```python
from build123d import *

# Parameters (mm, degrees)
CUT_EXTRUDE1_DEPTH      = 296.465734054
CUT_EXTRUDE1_DEPTH_BACK = 296.465734054
SKETCH2_R               = 6.1


with BuildPart() as part:
    # Sketch1 → Revolve1 (revolve)
    with BuildSketch(Plane.XY):
        Polygon((-21.25, -80), (-21.25, -67), (-17.5, -67), (-17.5, 67), (-21.25, 67), (-21.25, 80), (-42.5, 80), (-125, 80), (-125, 70), (-125, -70), (-180, -70), (-180, -80), (-42.5, -80), align=None)
    revolve(axis=Axis((0, 80, 0), (0, -1, 0)))

    # Sketch2 → Cut-Extrude1 (cut, two sides: drawn at the far end of the back side and taken through both)
    with BuildSketch(Plane(origin=(0, -70, 0), x_dir=(1, 0, 0), z_dir=(0, 1, 0)).offset(-CUT_EXTRUDE1_DEPTH_BACK)):
        with Locations(Location((0, 150, 0), (0, 0, 270))):
            Circle(SKETCH2_R)
        with Locations(Location((57.402514855, 138.581929877, 0), (0, 0, 270))):
            Circle(SKETCH2_R)
        with Locations(Location((106.066017178, 106.066017178, 0), (0, 0, 270))):
            Circle(SKETCH2_R)
        with Locations(Location((138.581929877, 57.402514855, 0), (0, 0, 270))):
            Circle(SKETCH2_R)
        with Locations(Location((150, 0, 0), (0, 0, 270))):
            Circle(SKETCH2_R)
        with Locations(Location((138.581929877, -57.402514855, 0), (0, 0, 270))):
            Circle(SKETCH2_R)
        with Locations(Location((106.066017178, -106.066017178, 0), (0, 0, 270))):
            Circle(SKETCH2_R)
        with Locations(Location((57.402514855, -138.581929877, 0), (0, 0, 270))):
            Circle(SKETCH2_R)
        with Locations(Location((0, -150, 0), (0, 0, 270))):
            Circle(SKETCH2_R)
        with Locations(Location((-57.402514855, -138.581929877, 0), (0, 0, 270))):
            Circle(SKETCH2_R)
        with Locations(Location((-106.066017178, -106.066017178, 0), (0, 0, 270))):
            Circle(SKETCH2_R)
        with Locations(Location((-138.581929877, -57.402514855, 0), (0, 0, 270))):
            Circle(SKETCH2_R)
        with Locations(Location((-150, 0, 0), (0, 0, 270))):
            Circle(SKETCH2_R)
        with Locations(Location((-138.581929877, 57.402514855, 0), (0, 0, 270))):
            Circle(SKETCH2_R)
        with Locations(Location((-106.066017178, 106.066017178, 0), (0, 0, 270))):
            Circle(SKETCH2_R)
        with Locations(Location((-57.402514855, 138.581929877, 0), (0, 0, 270))):
            Circle(SKETCH2_R)
    extrude(amount=CUT_EXTRUDE1_DEPTH + CUT_EXTRUDE1_DEPTH_BACK, mode=Mode.SUBTRACT)


solid = part.part
```
Read the model definition and answer for the solid it produces. Units are mm, in the model's axes. A direction names the side the tool comes from. Give positions to 0.01 mm unless a question says otherwise; leave off trailing zeros. Write each loop counter-clockwise with the first axis right and the second up, starting at its lowest first coordinate (ties: lowest second). Pieces come first, ordered by that corner, then holes. Notation, with made-up numbers: (75, 34) -> (114, 34) arc R25 ccw to (114, 52) -> close; hole circle Ø7 at (-25, 17). An arc over 180 degrees is marked (long way). Answer in a Markdown table with one row per item.
1) Determine the mould class of faces 4 (the cylindrical face through (16.863, 73.591, 12.93)), 5 (the cylindrical face through (144.045, -75.07, -1.322)), 6 (the flat face through (-2, 80, 26)), 7 (the cylindrical face through (-83.06, -75.07, 159.69)) for opening direction X: released by +X, released by -X, zero draft, split by the parting line, or undercut.
Results list:
| item | result |
|---|---|
| face 4 | undercut |
| face 5 | undercut |
| face 6 | zero draft |
| face 7 | split by the parting line |
2) Section A-A on z = 0 is taken. Give the vertices of the cut face in (x, y), plus the area to 3 significant figures.
Results list:
| item | result |
|---|---|
| outline | (-180, -80) -> (-156.1, -80) -> (-156.1, -70) -> (-180, -70) -> close; (-143.9, -80) -> (-21.25, -80) -> (-21.25, -67) -> (-17.5, -67) -> (-17.5, 67) -> (-21.25, 67) -> (-21.25, 80) -> (-125, 80) -> (-125, -70) -> (-143.9, -70) -> close; (17.5, -67) -> (21.25, -67) -> (21.25, -80) -> (143.9, -80) -> (143.9, -70) -> (125, -70) -> (125, 80) -> (21.25, 80) -> (21.25, 67) -> (17.5, 67) -> close; (156.1, -80) -> (180, -80) -> (180, -70) -> (156.1, -70) -> close |
| area | 35,100 mm^2 |
3) A tool of negligible diameter and unlimited length cuts with its end or side. For faces 1 (the flat face through (-3, -67, -17.4)), 2 (the flat face through (-123, -70, 37)), 3 (the cylindrical face through (0.268, -75.07, -156.094)), from which of +Z, -Z, +X, -X, +Y, -Y can it reach the whole face along a straight path? Write none if from no direction.
Results list:
| item | result |
|---|---|
| face 1 | -Y |
| face 2 | +Y |
| face 3 | +Y, -Y |
4) Each of these flat-tipped pins is pushed along its axis until it touches: pin 1 Ø12 at (y, z) = (-47.5, -99) entering from -X; pin 2 Ø3 at (x, y) = (113.5, 59) entering from -Z; pin 3 Ø1.5 at (y, z) = (-19.5, 43) entering from -X. Where does it stop, or does it pass through?
Results list:
| item | result |
|---|---|
| pin 1 | x = -83.52 |
| pin 2 | z = -55.51 |
| pin 3 | x = -117.64 |
5) Straight lines are drawn through the part: line 1 (X direction, y = -72.5, z = 0); line 2 (X direction, y = -37, z = 0). For each, find the intervals that lie inside material, in ascending order. Write a range as [from, to].
Results list:
| item | result |
|---|---|
| line 1 | [-180, -156.1], [-143.9, -21.25], [21.25, 143.9], [156.1, 180] |
| line 2 | [-125, -17.5], [17.5, 125] |
6) Section C-C on z = -150 is taken. Give the vertices of the cut face in (x, y), plus the area to 3 significant figures.
Results list:
| item | result |
|---|---|
| outline | (-99.5, -80) -> (-6.1, -80) -> (-6.1, -70) -> (-99.5, -70) -> close; (6.1, -80) -> (99.5, -80) -> (99.5, -70) -> (6.1, -70) -> close |
| area | 1,870 mm^2 |
7) Section B-B on x = 150 is taken. Give the vertices of the cut face in (y, z), plus the area to 3 significant figures.
Results list:
| item | result |
|---|---|
| outline | (-80, -99.5) -> (-70, -99.5) -> (-70, -6.1) -> (-80, -6.1) -> close; (-80, 6.1) -> (-70, 6.1) -> (-70, 99.5) -> (-80, 99.5) -> close |
| area | 1,870 mm^2 |
8) Section D-D on y = 51.5 is taken. Give the vertices of the cut face in (x, z), plus the area to 3 significant figures.
Results list:
| item | result |
|---|---|
| outline | circle Ø250 at (0, 0); hole circle Ø35 at (0, 0) |
| area | 48,100 mm^2 |
